Check sheet for the modelled part. Datum: model origin and axes. Units: mm. Face numbers are marked on the shaded views. A direction names the side the tool comes from. Give positions to 0.01 mm unless a question says otherwise; leave off trailing zeros. Write each loop counter-clockwise with the first axis right and the second up, starting at its lowest first coordinate (ties: lowest second). Pieces come first, ordered by that corner, then holes. Notation, with made-up numbers: M -23.5,43.25 L 3.5,43.25 A23 cw 3.5,76.25 Z; hole C 16,56 d7. An arc over 180 degrees is marked long. One line per item, written item: value. Start each with the question number.
from build123d import *

# Parameters (mm, degrees)
BASPROSKE_W         = 12
BASPROSKE_H         = 15
TOOTHCUT_DEPTH      = 25.372115214
TEETHCUTS_COUNT     = 18
TEETHCUTS_ANGLE     = 340
BORSKE_R            = 2.5
BORE_DEPTH          = 50.0000508
SKETCH_1_R          = 2.6
CUT_EXTRUDE_1_DEPTH = 25.269634752
EXTRUDE_2_DEPTH     = 12


with BuildPart() as part:
    # BasProSke → Base-Revolve (revolve)
    with BuildSketch(Plane(origin=(0, 0, 0), x_dir=(1, 0, 0), z_dir=(0, 1, 0)), mode=Mode.PRIVATE) as base_revolve_sk:
        with Locations((6, 7.5)):
            Rectangle(BASPROSKE_W, BASPROSKE_H)
    revolve(base_revolve_sk.sketch.rotate(Axis((-10, 0, 0), (1, 0, 0)), 180), axis=Axis((-10, 0, 0), (1, 0, 0)))

    # TooCutSke → ToothCut (cut, through all)
    with BuildSketch(Plane(origin=(0, 0, 0), x_dir=(0, 0, -1), z_dir=(1, 0, 0))):
        with BuildLine():
            ThreePointArc((0.759974923, 11.599129886), (0, 11.624), (-0.759974923, 11.599129886))
            ThreePointArc((-0.759974923, 11.599129886), (-1.229186471, 13.354767823), (-2.254227748, 14.855339189))
            ThreePointArc((-2.254227748, 14.855339189), (0, 15.0254), (2.254227748, 14.855339189))
            ThreePointArc((2.254227748, 14.855339189), (1.229186471, 13.354767823), (0.759974923, 11.599129886))
        make_face()
    toothcut = extrude(amount=TOOTHCUT_DEPTH, mode=Mode.SUBTRACT)

    # TeethCuts: ToothCut ×18 about axis
    teethcuts_axis = Axis((-10, 0, 0), (1, 0, 0))
    for i in range(1, TEETHCUTS_COUNT):
        add(toothcut.rotate(teethcuts_axis, i * TEETHCUTS_ANGLE / (TEETHCUTS_COUNT - 1)), mode=Mode.SUBTRACT)

    # BorSke → Bore (cut, symmetric)
    with BuildSketch(Plane(origin=(0, 0, 0), x_dir=(0, 0, -1), z_dir=(1, 0, 0))):
        with Locations(Location((0, 0, 0), (0, 0, 180))):
            Circle(BORSKE_R)
    extrude(amount=BORE_DEPTH, both=True, mode=Mode.SUBTRACT)

    # 草圖1 → 除料-伸長1 (cut, through all)
    with BuildSketch(Plane(origin=(12, 0, 0), x_dir=(0, 0, -1), z_dir=(1, 0, 0))):
        Circle(SKETCH_1_R)
    extrude(amount=-CUT_EXTRUDE_1_DEPTH, mode=Mode.SUBTRACT)

    # 草圖2 → 填料-伸長2 (add, through all)
    with BuildSketch(Plane(origin=(12, 0, 0), x_dir=(0, 0, -1), z_dir=(1, 0, 0))):
        with BuildLine():
            Line((0, 2.1), (1.532970972, 2.1))
            ThreePointArc((1.532970972, 2.1), (0, 2.6), (-1.532970972, 2.1))
            Line((-1.532970972, 2.1), (0, 2.1))
        make_face()
    extrude(amount=-EXTRUDE_2_DEPTH)


solid = part.part
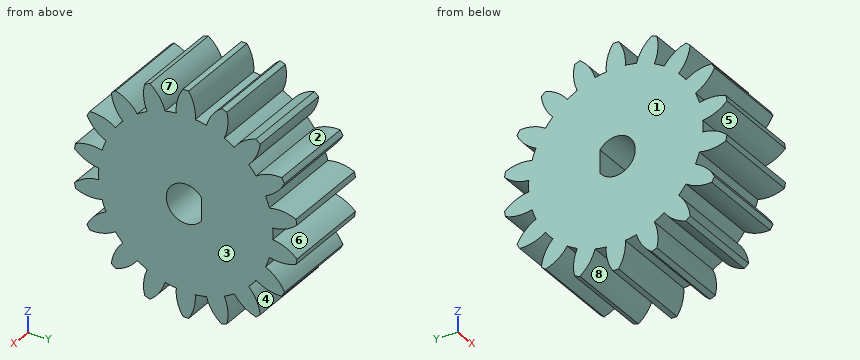
1) Material ranges on L1, parallel to Z at x = 8.75, y = 0; L2, parallel to Z at x = 2.75, y = 12.5; L3, parallel to Y at x = 1.25, z = 12, recorded low to high. Write a range as from..to.
2) Cross-section at D-D (z = -6.5). Record the boundary of the cut face in (x, y), plus the area to 3 significant figures.
3) Draft check along Z on the marked faces 6, 7 and 8. Enter one of: released by +Z, released by -Z, zero draft, split by the parting line, or undercut.
4) Gauge pin test, flat ends, axial feed: pin 1 (2 mm diameter, centred on x = 2.5, z = 11, fed in from +Y); pin 2 (4 mm diameter, centred on x = 6.5, z = -9.5, fed in from +Y); pin 3 (4 mm diameter, centred on x = 5.5, y = 2.5, fed in from -Z). Record the tip position at first contact, or that the pin passes through.
5) Cross-section at B-B (y = 0). Record the boundary of the cut face in (x, z).
6) Tool access check on the marked faces 1, 2, 3, 4 and 5. Record the directions out of +Z, -Z, +X, -X, +Y, -Y that give a thin tool (end or side, any length) a straight path to the whole face; none if there is none.
7) Cross-section at A-A (z = 0). Record the boundary of the cut face in (x, y).
8) Cross-section at C-C (z = -12.25). Record the boundary of the cut face in (x, y), plus the area to 3 significant figures.
Data:
1. L1: z = -15..-2.6, 2.6..15
1. L2: z = -7.84..-6.13, -3.43..-0.92, 0.92..3.43, 6.13..7.84
1. L3: y = -5.59..-3.01, -1.28..1.28, 3.01..5.59
2. outline: M 0,-12.78 L 12,-12.78 L 12,12.78 L 0,12.78 Z
2. area: 307 mm2
3. face 6: undercut
3. face 7: released by +Z
3. face 8: released by -Z
4. pin 1: stops at y = 9.93
4. pin 2: stops at y = 12.99
4. pin 3: stops at z = -14.8
5. outline: M 0,-15 L 12,-15 L 12,-2.6 L 0,-2.6 Z; M 0,2.6 L 12,2.6 L 12,15 L 0,15 Z
6. face 1: +Z, -Z, -X, +Y, -Y
6. face 2: +X, -X
6. face 3: +Z, -Z, +X, +Y, -Y
6. face 4: +X, -X, +Y
6. face 5: +X, -X, -Y
7. outline: M 0,-11.62 L 12,-11.62 L 12,-2.6 L 0,-2.6 Z; M 0,2.1 L 12,2.1 L 12,11.62 L 0,11.62 Z
8. outline: M 0,-5.62 L 12,-5.62 L 12,-3.13 L 0,-3.13 Z; M 0,-1.28 L 12,-1.28 L 12,1.28 L 0,1.28 Z; M 0,3.13 L 12,3.13 L 12,5.62 L 0,5.62 Z
8. area: 90.5 mm2
